Geometry check sheet. Reference: the model listing, model coordinates, mm. Face numbers are marked on the shaded views. A direction names the side the tool comes from. Give positions to 0.01 mm unless a question says otherwise; leave off trailing zeros. Order: outer loops, then holes, each group sorted by start corner. A loop starts at its lowest first (then second) coordinate and runs counter-clockwise, first axis right, second up. Notation, with made-up numbers: M 77,58.5 L 96,58.5 A22 cw 96,69.5 Z; hole C 35.5,44.5 d2. An arc over 180 degrees is marked long. Answer as a JSON object with one key per item and string values. Group by question number.
from build123d import *

# Parameters (mm, degrees)
RUNDUNG_DEPTH                   = 250
SKIZZE2_W                       = 22
SKIZZE2_H                       = 3.270726357
AUSSPARUNGLAUF_DEPTH            = 252.122480077
SKIZZE4_W                       = 20
SKIZZE4_H                       = 87.5
SCHNITT_LINEAR_AUSTRAGEN2_DEPTH = 252.164667101
SKIZZE5_R                       = 2.4
SCHNITT_LINEAR_AUSTRAGEN4_DEPTH = 6.4
SKIZZE6_R                       = 2.85
SCHNITT_LINEAR_AUSTRAGEN5_DEPTH = 1
SKIZZE9_W                       = 35
SKIZZE9_H                       = 6.605082277
AUFSATZ_LINEAR_AUSTRAGEN1_DEPTH = 24
SKIZZE10_W                      = 20
SKIZZE10_H                      = 8
SCHNITT_LINEAR_AUSTRAGEN7_DEPTH = 24
SCHNITT_LINEAR_AUSTRAGEN8_REACH = 277.025
SKIZZE11_R                      = 1.75
SKIZZE12_W                      = 45
SKIZZE12_H                      = 40
AUFSATZ_LINEAR_AUSTRAGEN2_DEPTH = 8
VERRUNDUNG1_R                   = 5
VERRUNDUNG6_R                   = 1
VERRUNDUNG7_R                   = 1
VERRUNDUNG8_R                   = 2


with BuildPart() as part:
    # Skizze1 → Rundung (new body)
    with BuildSketch(Plane(origin=(0, 0, 0), x_dir=(1, 0, 0), z_dir=(0, 1, 0))):
        with BuildLine():
            Line((-19.158288024, 7.5), (-22.5, 7.5))
            Line((-22.5, 7.5), (-22.5, -7.5))
            Line((-22.5, -7.5), (22.5, -7.5))
            Line((22.5, -7.5), (22.5, 7.5))
            Line((22.5, 7.5), (19.158288024, 7.5))
            ThreePointArc((19.158288024, 7.5), (0, 1.3), (-19.158288024, 7.5))
        make_face()
    extrude(amount=RUNDUNG_DEPTH)

    # Skizze2 → AussparungLauf (cut, through all)
    with BuildSketch(Plane(origin=(0, 250, 0), x_dir=(1, 0, 0), z_dir=(0, 1, 0))):
        with Locations((0, 2.935363178)):
            Rectangle(SKIZZE2_W, SKIZZE2_H)
    extrude(amount=-AUSSPARUNGLAUF_DEPTH, mode=Mode.SUBTRACT)

    # Skizze4 → Schnitt-Linear austragen2 (cut, through all)
    with BuildSketch(Plane(origin=(0, 0, -1.3), x_dir=(-1, 0, 0), z_dir=(0, 0, -1))):
        with Locations((0, 73.75)):
            Rectangle(SKIZZE4_W, SKIZZE4_H)
        with Locations((0, 176.25)):
            Rectangle(SKIZZE4_W, SKIZZE4_H)
    extrude(amount=-SCHNITT_LINEAR_AUSTRAGEN2_DEPTH, mode=Mode.SUBTRACT)

    # Skizze5 → Schnitt-Linear austragen4 (cut)
    with BuildSketch(Plane.XY.offset(7.5)):
        with Locations((-16, 32)):
            Circle(SKIZZE5_R)
        with Locations((16, 32)):
            Circle(SKIZZE5_R)
        with Locations((16, 48)):
            Circle(SKIZZE5_R)
        with Locations((16, 64)):
            Circle(SKIZZE5_R)
        with Locations((16, 80)):
            Circle(SKIZZE5_R)
        with Locations((-16, 48)):
            Circle(SKIZZE5_R)
        with Locations((-16, 64)):
            Circle(SKIZZE5_R)
        with Locations((-16, 80)):
            Circle(SKIZZE5_R)
    extrude(amount=-SCHNITT_LINEAR_AUSTRAGEN4_DEPTH, mode=Mode.SUBTRACT)

    # Skizze6 → Schnitt-Linear austragen5 (cut)
    with BuildSketch(Plane.XY.offset(1.1)):
        with Locations((-16, 32)):
            Circle(SKIZZE6_R)
        with Locations((16, 32)):
            Circle(SKIZZE6_R)
        with Locations((16, 48)):
            Circle(SKIZZE6_R)
        with Locations((16, 64)):
            Circle(SKIZZE6_R)
        with Locations((16, 80)):
            Circle(SKIZZE6_R)
        with Locations((-16, 48)):
            Circle(SKIZZE6_R)
        with Locations((-16, 64)):
            Circle(SKIZZE6_R)
        with Locations((-16, 80)):
            Circle(SKIZZE6_R)
    extrude(amount=-SCHNITT_LINEAR_AUSTRAGEN5_DEPTH, mode=Mode.SUBTRACT)

    # Skizze9 → Aufsatz-Linear austragen1 (add)
    with BuildSketch(Plane.XZ):
        with Locations((0, 4.197458862)):
            Rectangle(SKIZZE9_W, SKIZZE9_H)
    extrude(amount=AUFSATZ_LINEAR_AUSTRAGEN1_DEPTH)

    # Skizze10 → Schnitt-Linear austragen7 (cut)
    with BuildSketch(Plane.XY.offset(7.5)):
        with Locations((0, -12)):
            Rectangle(SKIZZE10_W, SKIZZE10_H)
    extrude(amount=-SCHNITT_LINEAR_AUSTRAGEN7_DEPTH, mode=Mode.SUBTRACT)

    # Skizze11 → Schnitt-Linear austragen8 (cut, up to next)
    with BuildSketch(Plane.XZ.offset(24), mode=Mode.PRIVATE) as schnitt_linear_austragen8_sk1:
        with Locations(Location((-5, 4.197458861, 0), (0, 0, 270))):
            Circle(SKIZZE11_R)
    schnitt_linear_austragen8_tool1 = extrude(schnitt_linear_austragen8_sk1.sketch, amount=-SCHNITT_LINEAR_AUSTRAGEN8_REACH, mode=Mode.PRIVATE) & part.part
    # Skizze11 → Schnitt-Linear austragen8 (cut, up to next)
    with BuildSketch(Plane.XZ.offset(24), mode=Mode.PRIVATE) as schnitt_linear_austragen8_sk2:
        with Locations((5, 4.197458861)):
            Circle(SKIZZE11_R)
    schnitt_linear_austragen8_tool2 = extrude(schnitt_linear_austragen8_sk2.sketch, amount=-SCHNITT_LINEAR_AUSTRAGEN8_REACH, mode=Mode.PRIVATE) & part.part
    add(schnitt_linear_austragen8_tool1.solids().sort_by_distance((-5, -24, 4.197459))[0], mode=Mode.SUBTRACT)
    add(schnitt_linear_austragen8_tool2.solids().sort_by_distance((5, -24, 4.197459))[0], mode=Mode.SUBTRACT)

    # Skizze12 → Aufsatz-Linear austragen2 (add)
    with BuildSketch(Plane(origin=(0, 250, 0), x_dir=(1, 0, 0), z_dir=(0, 1, 0))):
        with Locations((0, 12.5)):
            Rectangle(SKIZZE12_W, SKIZZE12_H)
    extrude(amount=AUFSATZ_LINEAR_AUSTRAGEN2_DEPTH)

    # Verrundung1
    verrundung1_edges = [part.edges().sort_by_distance(p)[0] for p in [
        (10, 132.5, 3.1),
        (10, 220, 3.1),
        (-10, 220, 3.1),
        (-10, 132.5, 3.1),
        (10, 30, 3.1),
        (10, 117.5, 3.1),
        (-10, 117.5, 3.1),
        (-10, 30, 3.1),
    ]]
    fillet(verrundung1_edges, radius=VERRUNDUNG1_R)

    # Verrundung6
    verrundung6_edges = [part.edges().sort_by_distance(p)[0] for p in [
        (-20.829144012, 250, -7.5),
        (15.231246671, 250, -5.063878545),
        (0, 250, -1.3),
        (11, 250, -2.252841171),
        (-11, 125, -3.205682342),
        (-11, 250, -2.252841171),
        (20.829144012, 250, -7.5),
        (-15.231246671, 250, -5.063878545),
    ]]
    fillet(verrundung6_edges, radius=VERRUNDUNG6_R)

    # Verrundung7
    verrundung7_edges = [part.edges().sort_by_distance(p)[0] for p in [
        (0, 250, -32.5),
        (22.5, 254, -32.5),
        (-22.5, 250, -20.5),
        (-22.5, 254, -32.5),
        (22.5, 258, -12.5),
        (0, 258, -32.5),
        (-22.5, 258, -12.5),
        (22.5, 250, -20.5),
        (22.5, 124.5, -7.5),
        (-22.5, 124.5, -7.5),
        (22.5, 249.707106781, -7.792893219),
        (-22.5, 249.707106781, -7.792893219),
    ]]
    fillet(verrundung7_edges, radius=VERRUNDUNG7_R)

    # Verrundung8
    verrundung8_edges = [part.edges().sort_by_distance(p)[0] for p in [
        (-17.5, -24, 4.197458861),
        (17.5, -24, 4.197458861),
    ]]
    fillet(verrundung8_edges, radius=VERRUNDUNG8_R)


solid = part.part
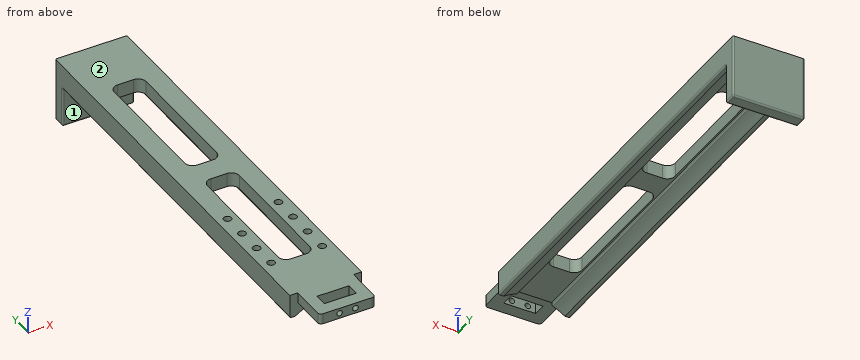
1. Thickness scan on line 1 along X through (y, z) = (80, 0); line 2 along Z through (x, y) = (5, -20); line 3 along Z through (x, y) = (-4, 245). Record the ranges inside material, lowest first. Write a range as [from, to].
2. Cross-section at C-C (y = 93). Record the cut outline in (x, z), and give its area (3 significant figures).
3. Access from +Z, -Z, +X, -X, +Y, -Y to the whole of each face (thin tool, end or side, straight path). Record for the marked faces 1 and 2.
4. Depth check by flat-ended pin: pin 1 (3.5 mm diameter, centred on y = -14.5, z = 4.5, fed in from +X); pin 2 (1.7 mm diameter, centred on x = 16.5, y = 33.5, fed in from -Z); pin 3 (3 mm diameter, centred on x = -15, y = 81, fed in from -Z); pin 4 (12 mm diameter, centred on y = 168, z = -15.5, fed in from +X). Enter the tip coordinate at first touch or a pass-through.
5. Cross-section at B-B (z = -17). Record the cut outline in (x, y).
Report:
{
 "1": {"line 1": "x = [-22.5, -10], [10, 22.5]", "line 2": "z = [0.89, 2.45], [5.95, 7.5]", "line 3": "z = [-1.3, 7.5]"},
 "2": {"outline": "M -22.5,-6.5 A1 ccw -21.5,-7.5 L -19.16,-7.5 A32.7 cw -11.64,-3.44 A1 ccw -11,-2.51 L -11,-1.3 L -10,-1.3 L -10,7.5 L -22.5,7.5 Z; M 10,-1.3 L 11,-1.3 L 11,-3.21 A32.7 cw 19.16,-7.5 L 21.5,-7.5 A1 ccw 22.5,-6.5 L 22.5,7.5 L 10,7.5 Z", "area": "323 mm2"},
 "3": {"face 1": "-Z, -Y", "face 2": "+Z, +X, -X, +Y, -Y"},
 "4": {"pin 1": "stops at x = 17.5", "pin 2": "stops at z = -6.28", "pin 3": "stops at z = -5.77", "pin 4": "passes through"},
 "5": {"outline": "M -22.5,251 A1 ccw -21.5,250 L 21.5,250 A1 ccw 22.5,251 L 22.5,257 A1 ccw 21.5,258 L -21.5,258 A1 ccw -22.5,257 Z"}
}
